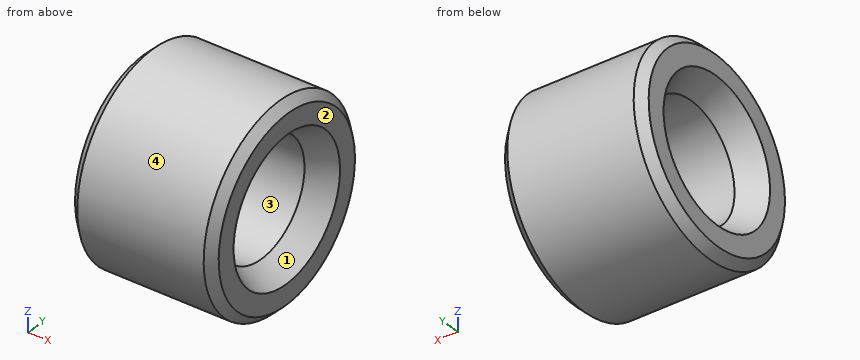
from build123d import *

# Parameters (mm, degrees)
SKETCH1_W     = 5
SKETCH1_H     = 1.5
CHAMFER1_SIZE = 0.3


with BuildPart() as part:
    # Sketch1 → Revolve1 (revolve)
    with BuildSketch(Plane.XY, mode=Mode.PRIVATE) as revolve1_sk:
        with Locations((2.5, 2.75)):
            Rectangle(SKETCH1_W, SKETCH1_H)
    revolve(revolve1_sk.sketch.rotate(Axis((0, 0, 0), (1, 0, 0)), 90), axis=Axis((0, 0, 0), (1, 0, 0)))

    # Chamfer1
    chamfer1_edges = [part.edges().sort_by_distance(p)[0] for p in [
        (5, 0, -3.5),
        (0, 0, -3.5),
    ]]
    chamfer(chamfer1_edges, length=CHAMFER1_SIZE)

    # Sketch2 → Cut-Revolve1 (revolve, cut)
    with BuildSketch(Plane.XY, mode=Mode.PRIVATE) as cut_revolve1_sk:
        Polygon((0, 2.5), (0, 2), (0.866025404, 2), align=None)
        Polygon((4.133974596, 2), (5, 2.5), (5, 2), align=None)
    revolve(cut_revolve1_sk.sketch.rotate(Axis((0, 0, 0), (1, 0, 0)), 90), axis=Axis((0, 0, 0), (1, 0, 0)), mode=Mode.SUBTRACT)


solid = part.part
Input: part model. Units: mm. Frame: model coordinates. Face numbers are marked on the shaded views. Coordinates: 2 decimals unless noted, no trailing zeros. Loops run counter-clockwise (first coordinate to the right, second up) from the corner with the lowest first, then second, coordinate; pieces in that order, holes last.
Q1. Cut plane C-C (x = 2.4). Output: boundary loops of the cut face in (y, z).
Q2. Material intervals for line 1 (Y direction, x = 2.1, z = 0); line 2 (Y direction, x = 4.5, z = -0.5); line 3 (Z direction, x = 2.05, y = -0.5), sorted ascending.
Q3. Draft query along Y for the marked faces 1, 2, 3 and 4. Return one class per face: +Y half, -Y half, draft (parallel to the pull), parting line (faces both ways), or undercut.
Q4. Cut plane A-A (z = 0). Output: boundary loops of the cut face in (x, y), then the cut area to 3 significant figures.
Q5. Contact query for flat-ended pins moving along their axis: pin 1 (3 mm diameter, centred on y = 1, z = -0.5, fed in from +X); pin 2 (2 mm diameter, centred on y = 1, z = -0.5, fed in from +X); pin 3 (2 mm diameter, centred on x = 3.5, y = -2.5, fed in from +Z); pin 4 (2 mm diameter, centred on x = 1, z = 2.5, fed in from +Y). Output: stop coordinate, or through.
Working result:
1. outline: circle Ø7 at (0, 0); hole circle Ø4 at (0, 0)
2. line 1: y = -3.5 to -2, 2 to 3.5
2. line 2: y = -3.46 to -2.15, 2.15 to 3.46
2. line 3: z = -3.46 to -1.94, 1.94 to 3.46
3. face 1: undercut
3. face 2: draft
3. face 3: undercut
3. face 4: parting line
4. outline: (0, -3.2) - (0.3, -3.5) - (4.7, -3.5) - (5, -3.2) - (5, -2.5) - (4.13, -2) - (0.87, -2) - (0, -2.5) - close; (0, 2.5) - (0.87, 2) - (4.13, 2) - (5, 2.5) - (5, 3.2) - (4.7, 3.5) - (0.3, 3.5) - (0, 3.2) - close
4. area: 14.0 mm2
5. pin 1: stops at x = 5
5. pin 2: stops at x = 4.34
5. pin 3: stops at z = 3.16
5. pin 4: stops at y = 3.16
